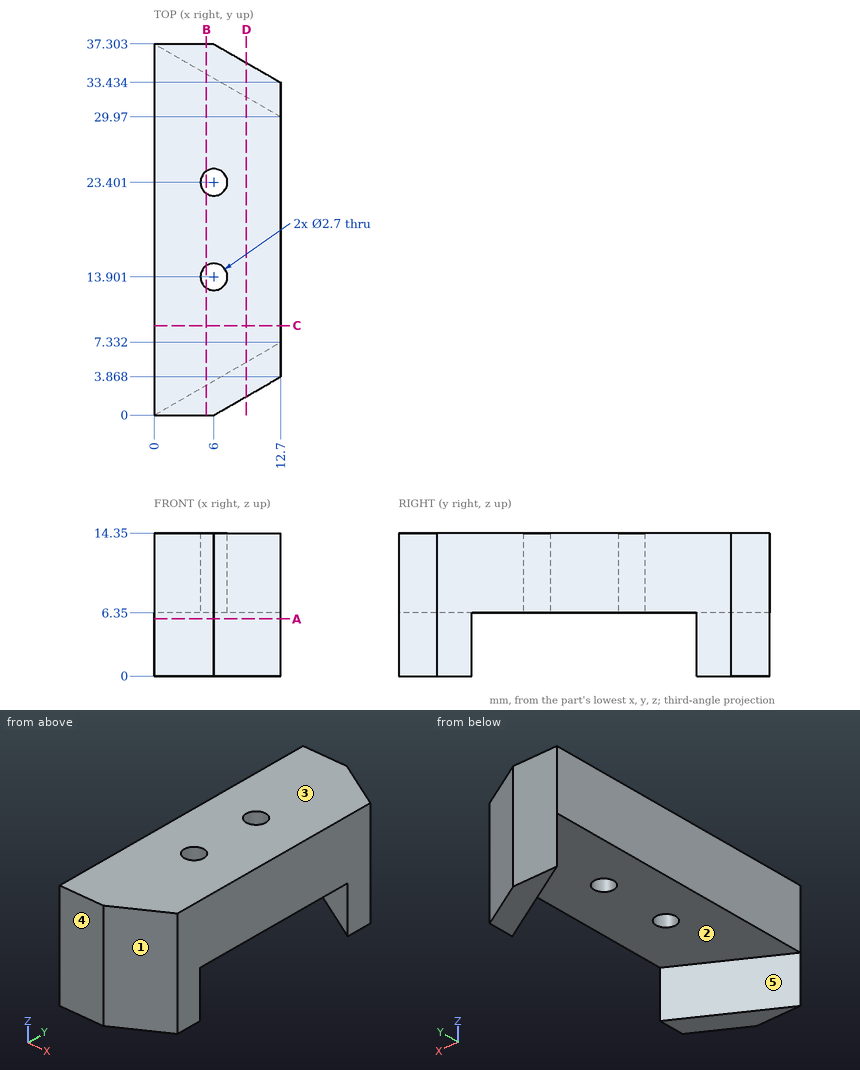
Source: three-view drawing plus pictorial views. Frame: mm from the lowest corner of the part. A direction names the side the tool comes from. Give positions to 0.01 mm unless a question says otherwise; leave off trailing zeros. Order: outer loops, then holes, each group sorted by start corner. A loop starts at its lowest first (then second) coordinate and runs counter-clockwise, first axis right, second up. Notation, with made-up numbers: M 17,-9.75 L 26,-9.75 A22 ccw 26,10.25 Z; hole C 75,45.5 d11. An arc over 180 degrees is marked long. One line per question, with ' | ' between items. Start each with the question number.
1. Material intervals for probe 1 along Y at (x, z) = (6, 10); probe 2 along Z at (x, y) = (8.5, 30.5); probe 3 along Y at (x, z) = (8.5, 3.25) (1 decimal), sorted ascending. Write a range as [from, to].
2. First-contact query: pin 1 Ø4.5 at (x, y) = (6, 23.4) entering from -Z; pin 2 Ø3 at (x, z) = (10, 5.5) entering from +Y; pin 3 Ø3 at (x, z) = (5, 2) entering from -Y; pin 4 Ø1 at (x, z) = (9, 11.5) entering from -Y. Flat tips, straight axial feed; report the tip coordinate or a pass-through.
3. Access query for the marked faces 4 and 5. Directions: +Z, -Z, +X, -X, +Y, -Y. A direction counts if a zero-diameter tool reaches every point of the face in a straight line with its end or side. Return the directions, or none.
4. Section query C-C (y = 9). Return the cut outline in (x, z), and give its area (3 significant figures).
5. Section query A-A (z = 5.75). Return the cut outline in (x, y) (1 decimal).
6. Section query D-D (x = 9.25). Return the cut outline in (y, z).
7. Section query B-B (x = 5.25). Return the cut outline in (y, z), and give its area (3 significant figures).
8. Pull-direction query (Y, two-part tool) for the marked faces 1, 2 and 3; classes: released by +Y, released by -Y, zero draft, split by the parting line, or undercut.
Here are the results:
1) probe 1: [0, 12.55], [15.25, 22.05], [24.75, 37.3] | probe 2: [6.35, 14.35] | probe 3: [1.4, 4.9], [32.4, 35.9]
2) pin 1: z = 6.35 | pin 2: y = 35.86 | pin 3: y = 0 | pin 4: y = 1.44
3) face 4: +Z, -Z, +X, -X, -Y | face 5: -Z, -X
4) outline: M 0,6.35 L 12.7,6.35 L 12.7,14.35 L 0,14.35 Z | area: 102 mm²
5) outline: M 0,0 L 6,0 L 12.7,3.9 L 12.7,7.3 Z; M 0,37.3 L 12.7,30 L 12.7,33.4 L 6,37.3 Z
6) outline: M 1.88,0 L 5.34,0 L 5.34,6.35 L 31.96,6.35 L 31.96,0 L 35.43,0 L 35.43,14.35 L 1.88,14.35 Z
7) outline: M 0,0 L 3.03,0 L 3.03,6.35 L 12.78,6.35 L 12.78,14.35 L 0,14.35 Z; M 15.02,6.35 L 22.28,6.35 L 22.28,14.35 L 15.02,14.35 Z; M 24.52,6.35 L 34.27,6.35 L 34.27,0 L 37.3,0 L 37.3,14.35 L 24.52,14.35 Z | area: 301 mm²
8) face 1: released by -Y | face 2: undercut | face 3: zero draft
